Job drawing, mm, ordinate dimensions from the low corner. One solid piece. A direction names the side the tool comes from. Coordinates: 2 decimals unless noted, no trailing zeros. Order: outer loops, then holes, each group sorted by start corner. A loop starts at its lowest first (then second) coordinate and runs counter-clockwise, first axis right, second up. Notation, with made-up numbers: M -22,52.5 L -9,52.5 A17 cw -9,69.5 Z; hole C 60,-17.75 d9. An arc over 180 degrees is marked long. Write item = value, one per line. Start each with the question number.
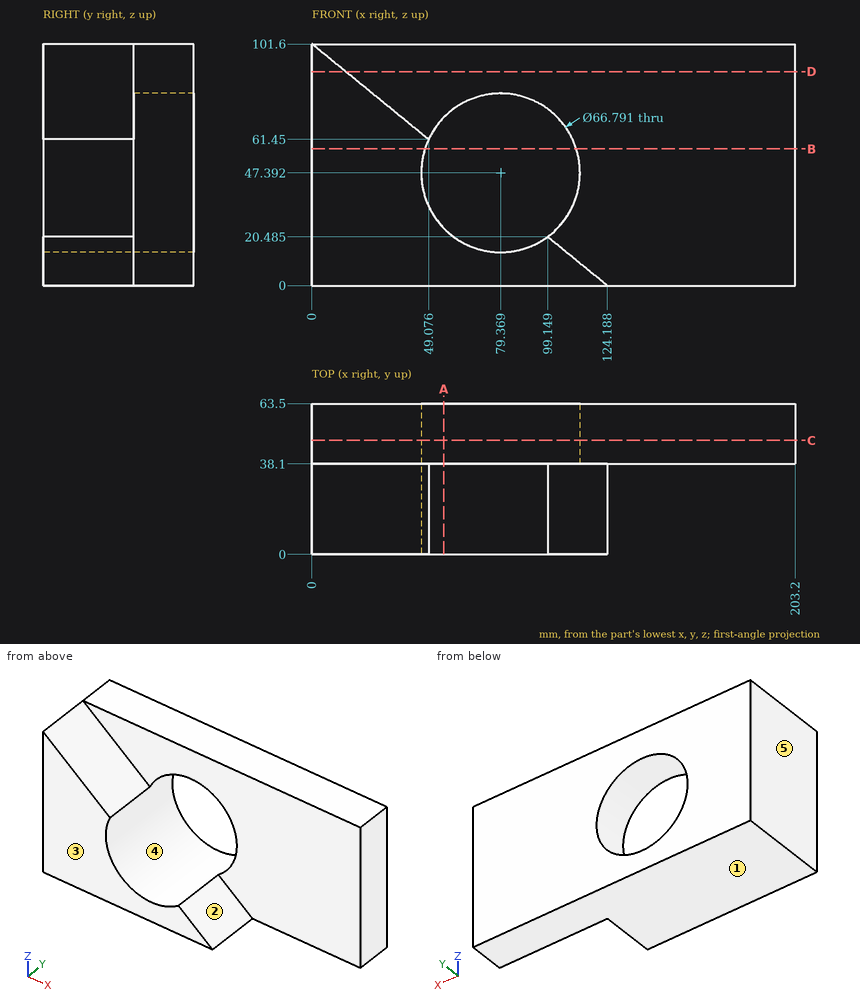
Item 1: Pull direction X, two halves, no side cores. Call the marked faces 3, 4 and 5: pulls with the +X half, pulls with the -X half, needs draft (parallel to the pull), parting line crosses it, or undercut.
Item 2: Wall check: line 1 along Y through (x, z) = (141.5, 94.5); line 2 along X through (y, z) = (39, 65.5); line 3 along Z through (x, y) = (99.5, 55) (1 decimal). Give the ranges that are in metal, low to high. Write a range as [from, to].
Item 3: Cut at D-D, the plane z = 90. Write the cut outline in (x, y).
Item 4: Cut at A-A, the plane x = 55.5. Write the cut outline in (y, z) (1 decimal), and give its area (3 significant figures).
Item 5: Cut at C-C, the plane y = 48. Write the cut outline in (x, z) (1 decimal).
Item 6: Cut at B-B, the plane z = 57.5. Write the cut outline in (x, y).
Item 7: Flat gauge pins, fed straight in: pin 1 (5 mm diameter, centred on y = 21.5, z = 79, fed in from +X); pin 2 (3 mm diameter, centred on x = 81.5, y = 32, fed in from +Z); pin 3 (10 mm diameter, centred on x = 161, z = 60, fed in from -Y). Where does each tip first touch, or does it go through?
Item 8: 3-axis set-ups, long thin cutter, end or side, ignore diameter. For the marked faces 1 and 2: which of +Z, -Z, +X, -X, +Y, -Y reach the whole face in a straight line?
Filled sheet:
q1.face_3 = needs draft
q1.face_4 = undercut
q1.face_5 = pulls with the -X half
q2.line_1 = [38.1, 63.5]
q2.line_2 = [0, 51.31], [107.43, 203.2]
q2.line_3 = [0, 20.7], [74, 101.6]
q3.outline = M 0,0 L 14.18,0 L 14.18,38.1 L 203.2,38.1 L 203.2,63.5 L 0,63.5 Z
q4.outline = M 0,0 L 63.5,0 L 63.5,24 L 0,24 Z; M 38.1,70.7 L 63.5,70.7 L 63.5,101.6 L 38.1,101.6 Z
q4.area = 2,310 mm2
q5.outline = M 0,0 L 203.2,0 L 203.2,101.6 L 0,101.6 Z; hole C 79.4,47.4 d66.8
q6.outline = M 0,0 L 47.54,0 L 47.54,63.5 L 0,63.5 Z; M 111.2,38.1 L 203.2,38.1 L 203.2,63.5 L 111.2,63.5 Z
q7.pin_1 = 30.68
q7.pin_2 = 14.19
q7.pin_3 = 38.1
q8.face_1 = -Z, +X, -X, +Y, -Y
q8.face_2 = +Z, +X, -Y
